Model file for the job. Use its own axes, mm. Face numbers are marked on the shaded views. A direction names the side the tool comes from. Round coordinates to 2 decimals unless told otherwise and drop trailing zeros. Loops run counter-clockwise (first coordinate to the right, second up) from the corner with the lowest first, then second, coordinate; pieces in that order, holes last. Notation, with made-up numbers: M 32,28.5 L 47,28.5 A7 cw 47,40.5 Z; hole C -32,-40 d5. An arc over 180 degrees is marked long. Use a Markdown table: item, result. Add a question column.
Item 1: Saw through at A-A on y = 49. Write the cut outline in (x, z), then the cut area to 3 significant figures.
Item 2: Tool access for the marked faces 1 and 2: list every direction of +Z, -Z, +X, -X, +Y, -Y with a clear straight run to the whole face (end or side of a thin tool).
Item 3: Pin check, flat tips, straight feed: P1, Ø8, axis at x = 17, y = 111.5, coming from the -Z side; P2, Ø5, axis at y = 54.5, z = -24.5, coming from the -X side; P3, Ø4, axis at x = 0.5, y = 61.5, coming from the +Z side. Stop position of each tip, or through.
Item 4: Wall check: L1, parallel to X at y = 104, z = 12; L2, parallel to X at y = 91, z = 4; L3, parallel to Z at x = -29.5, y = 108. Give the ranges that are in metal, low to high. Write a range as from..to.
Item 5: Two-plate mould, pull along X, no slides. Class the marked faces 3, 4 and 5: +X half, -X half, draft (parallel to the pull), parting line (faces both ways), or undercut.
```python
from build123d import *

# Parameters (mm, degrees)
SKETCH3_R           = 25
CUT_EXTRUDE1_DEPTH  = 129.210764141
SKETCH4_R           = 35
CUT_EXTRUDE2_DEPTH  = 10
FILLET1_R           = 15
SKETCH5_W           = 51
SKETCH5_H           = 51
CUT_EXTRUDE3_DEPTH  = 129.210764141
BOSS_EXTRUDE1_DEPTH = 10
CUT_EXTRUDE4_DEPTH  = 10
FILLET2_R           = 5


with BuildPart() as part:
    # Sketch2 → Loft1 section 0
    with BuildSketch(Plane(origin=(0, 53, 0), x_dir=(1, 0, 0), z_dir=(0, 1, 0))):
        with BuildLine():
            Line((-29.0467, -29.0467), (29.0467, -29.0467))
            Line((29.0467, -29.0467), (29.0467, 29.0467))
            Line((29.0467, 29.0467), (-29.0467, 29.0467))
            Line((-29.0467, 29.0467), (-29.0467, -29.0467))
        make_face()
    # Sketch1 → Loft1 section 1
    with BuildSketch(Plane(origin=(0, 0, 0), x_dir=(1, 0, 0), z_dir=(0, 1, 0))):
        with BuildLine():
            Line((-51, -51), (51, -51))
            Line((51, -51), (51, 51))
            Line((51, 51), (-51, 51))
            Line((-51, 51), (-51, -51))
        make_face()
    loft1 = loft()

    # Mirror1: Loft1 across plane
    add(loft1.mirror(Plane.ZX.offset(53)))

    # Sketch3 → Cut-Extrude1 (cut, through all)
    with BuildSketch(Plane(origin=(0, 106, 0), x_dir=(1, 0, 0), z_dir=(0, 1, 0))):
        with Locations(Location((0, 0, 0), (0, 0, 270))):
            Circle(SKETCH3_R)
    extrude(amount=-CUT_EXTRUDE1_DEPTH, mode=Mode.SUBTRACT)

    # Sketch4 → Cut-Extrude2 (cut)
    with BuildSketch(Plane(origin=(0, 106, 0), x_dir=(1, 0, 0), z_dir=(0, 1, 0))):
        with Locations(Location((0, 0, 0), (0, 0, 270))):
            Circle(SKETCH4_R)
    cut_extrude2 = extrude(amount=-CUT_EXTRUDE2_DEPTH, mode=Mode.SUBTRACT)

    # Mirror2: Cut-Extrude2 across plane
    add(cut_extrude2.mirror(Plane.ZX.offset(53)), mode=Mode.SUBTRACT)

    # Fillet1
    # the kernel refuses this fillet: 15 mm, written as the material it adds along each edge
    with BuildSketch(Plane(origin=(44.579695283, 53, -29.0467), x_dir=(0, -0.923879648411862, -0.38268315255622926), z_dir=(-1, 0, 0))) as fillet1_piece_1_section:
        with BuildLine():
            CenterArc((FILLET1_R * 0.414213207547, -FILLET1_R), FILLET1_R, 90, 44.999965294)
            Line((-FILLET1_R * 0.292893145326, -FILLET1_R * 0.292892790501), (0, 0))
            Line((0, 0), (FILLET1_R * 0.414213207547, 0))
        make_face()
    fillet1_piece_1 = extrude(amount=89.159390566, mode=Mode.PRIVATE)
    fillet1_piece_1 = fillet1_piece_1 - Plane(origin=(-45.282580968, 53, -29.0467), x_dir=(0.9238796484118622, -0.3826831525562288, 0), z_dir=(0, 0, -1)) * Cylinder(15, 204, mode=Mode.PRIVATE)
    fillet1_piece_1 = fillet1_piece_1 - Plane(origin=(45.282580968, 53, -29.0467), x_dir=(-0.9238796484118622, -0.3826831525562288, 0), z_dir=(0, 0, 1)) * Cylinder(15, 204, mode=Mode.PRIVATE)
    add(fillet1_piece_1)
    with BuildSketch(Plane(origin=(-29.0467, 53, -44.579695283), x_dir=(-0.3826831525562283, -0.9238796484118624, 0), z_dir=(0, 0, 1))) as fillet1_piece_2_section:
        with BuildLine():
            CenterArc((FILLET1_R * 0.414213207547, -FILLET1_R), FILLET1_R, 90, 44.999965294)
            Line((-FILLET1_R * 0.292893145326, -FILLET1_R * 0.292892790501), (0, 0))
            Line((0, 0), (FILLET1_R * 0.414213207547, 0))
        make_face()
    fillet1_piece_2 = extrude(amount=89.159390566, mode=Mode.PRIVATE)
    fillet1_piece_2 = fillet1_piece_2 - Plane(origin=(-29.0467, 53, 45.282580968), x_dir=(0, -0.3826831525562288, -0.9238796484118622), z_dir=(-1, 0, 0)) * Cylinder(15, 204, mode=Mode.PRIVATE)
    fillet1_piece_2 = fillet1_piece_2 - Plane(origin=(-29.0467, 53, -45.282580968), x_dir=(0, -0.3826831525562288, 0.9238796484118622), z_dir=(1, 0, 0)) * Cylinder(15, 204, mode=Mode.PRIVATE)
    add(fillet1_piece_2)
    with BuildSketch(Plane(origin=(-44.579695283, 53, 29.0467), x_dir=(0, -0.923879648411862, 0.38268315255622926), z_dir=(1, 0, 0))) as fillet1_piece_3_section:
        with BuildLine():
            CenterArc((FILLET1_R * 0.414213207547, -FILLET1_R), FILLET1_R, 90, 44.999965294)
            Line((-FILLET1_R * 0.292893145326, -FILLET1_R * 0.292892790501), (0, 0))
            Line((0, 0), (FILLET1_R * 0.414213207547, 0))
        make_face()
    fillet1_piece_3 = extrude(amount=89.159390566, mode=Mode.PRIVATE)
    fillet1_piece_3 = fillet1_piece_3 - Plane(origin=(-45.282580968, 53, 29.0467), x_dir=(0.9238796484118622, -0.3826831525562288, 0), z_dir=(0, 0, -1)) * Cylinder(15, 204, mode=Mode.PRIVATE)
    fillet1_piece_3 = fillet1_piece_3 - Plane(origin=(45.282580968, 53, 29.0467), x_dir=(-0.9238796484118622, -0.3826831525562288, 0), z_dir=(0, 0, 1)) * Cylinder(15, 204, mode=Mode.PRIVATE)
    add(fillet1_piece_3)
    with BuildSketch(Plane(origin=(29.0467, 53, 44.579695283), x_dir=(0.3826831525562283, -0.9238796484118624, 0), z_dir=(0, 0, -1))) as fillet1_piece_4_section:
        with BuildLine():
            CenterArc((FILLET1_R * 0.414213207547, -FILLET1_R), FILLET1_R, 90, 44.999965294)
            Line((-FILLET1_R * 0.292893145326, -FILLET1_R * 0.292892790501), (0, 0))
            Line((0, 0), (FILLET1_R * 0.414213207547, 0))
        make_face()
    fillet1_piece_4 = extrude(amount=89.159390566, mode=Mode.PRIVATE)
    fillet1_piece_4 = fillet1_piece_4 - Plane(origin=(29.0467, 53, 45.282580968), x_dir=(0, -0.3826831525562288, -0.9238796484118622), z_dir=(-1, 0, 0)) * Cylinder(15, 204, mode=Mode.PRIVATE)
    fillet1_piece_4 = fillet1_piece_4 - Plane(origin=(29.0467, 53, -45.282580968), x_dir=(0, -0.3826831525562288, 0.9238796484118622), z_dir=(1, 0, 0)) * Cylinder(15, 204, mode=Mode.PRIVATE)
    add(fillet1_piece_4)

    # Sketch5 → Cut-Extrude3 (cut, through all)
    with BuildSketch(Plane(origin=(0, 106, 0), x_dir=(1, 0, 0), z_dir=(0, 1, 0))):
        with Locations((25.5, 25.5)):
            Rectangle(SKETCH5_W, SKETCH5_H)
    extrude(amount=-CUT_EXTRUDE3_DEPTH, mode=Mode.SUBTRACT)

    # Sketch6 → Boss-Extrude1 (add)
    with BuildSketch(Plane(origin=(0, 106, 0), x_dir=(1, 0, 0), z_dir=(0, 1, 0))):
        Polygon((0, 51), (-51, 51), (-51, -51), (51, -51), (51, 0), (48, 0), (48, -48), (-48, -48), (-48, 48), (0, 48), align=None)
    extrude(amount=BOSS_EXTRUDE1_DEPTH)

    # Sketch7 → Cut-Extrude4 (cut)
    with BuildSketch(Plane(origin=(0, 106, 0), x_dir=(1, 0, 0), z_dir=(0, 1, 0))):
        with BuildLine():
            Line((-32.173358544, 27.930717857), (-42.779960262, 38.537319575))
            ThreePointArc((-42.779960262, 38.537319575), (-42.779960262, 42.779960262), (-38.537319575, 42.779960262))
            Line((-38.537319575, 42.779960262), (-27.930717857, 32.173358544))
            ThreePointArc((-27.930717857, 32.173358544), (-27.930717857, 27.930717857), (-32.173358544, 27.930717857))
        make_face()
        with BuildLine():
            Line((27.930717857, 32.173358544), (38.537319575, 42.779960262))
            ThreePointArc((38.537319575, 42.779960262), (42.779960262, 42.779960262), (42.779960262, 38.537319575))
            Line((42.779960262, 38.537319575), (32.173358544, 27.930717857))
            ThreePointArc((32.173358544, 27.930717857), (27.930717857, 27.930717857), (27.930717857, 32.173358544))
        make_face()
        with BuildLine():
            Line((32.173358544, -27.930717857), (42.779960262, -38.537319575))
            ThreePointArc((42.779960262, -38.537319575), (42.779960262, -42.779960262), (38.537319575, -42.779960262))
            Line((38.537319575, -42.779960262), (27.930717857, -32.173358544))
            ThreePointArc((27.930717857, -32.173358544), (27.930717857, -27.930717857), (32.173358544, -27.930717857))
        make_face()
        with BuildLine():
            Line((-27.930717857, -32.173358544), (-38.537319575, -42.779960262))
            ThreePointArc((-38.537319575, -42.779960262), (-42.779960262, -42.779960262), (-42.779960262, -38.537319575))
            Line((-42.779960262, -38.537319575), (-32.173358544, -27.930717857))
            ThreePointArc((-32.173358544, -27.930717857), (-27.930717857, -27.930717857), (-27.930717857, -32.173358544))
        make_face()
    extrude(amount=-CUT_EXTRUDE4_DEPTH, mode=Mode.SUBTRACT)

    # Fillet2
    fillet2_edges = [part.edges().sort_by_distance(p)[0] for p in [
        (-25.5, 106, -51),
        (-51, 106, 0),
        (51, 106, 25.5),
        (0, 106, 51),
    ]]
    fillet(fillet2_edges, radius=FILLET2_R)


solid = part.part
```
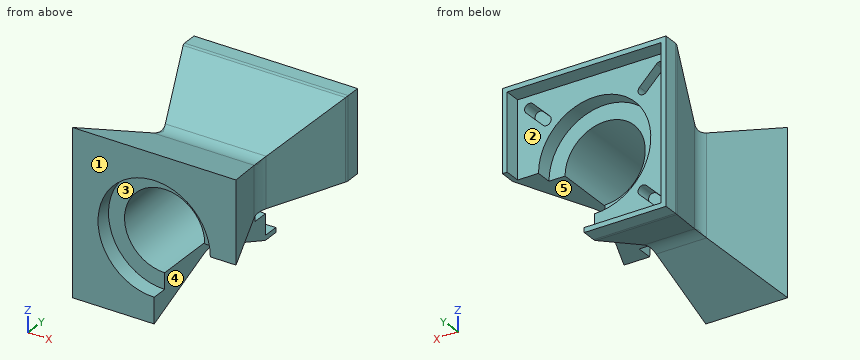
Entries:
| question | item | result |
|---|---|---|
| 1 | outline | M -30.83,-30.83 L 0,-30.83 L 0,-25 A25 cw long 25,0 L 30.83,0 L 30.83,30.83 L -30.83,30.83 Z |
| 1 | area | 1,380 mm2 |
| 2 | face 1 | +Z, -Z, +X, -X, -Y |
| 2 | face 2 | +Y |
| 3 | P1 | z = 48 |
| 3 | P2 | x = -30.83 |
| 3 | P3 | z = 33.4 |
| 4 | L1 | -50.17..-32.88, 32.88..50.17 |
| 4 | L2 | -44.79..-24.68, 24.68..44.79 |
| 4 | L3 | -51..-48, 48..51 |
| 5 | face 3 | undercut |
| 5 | face 4 | +X half |
| 5 | face 5 | draft |
